```python
from build123d import *

# Parameters (mm, degrees)
BOSS_EXTRUDE1_DEPTH = 15
SKETCH2_R           = 7.5
CUT_EXTRUDE1_DEPTH  = 15
SKETCH3_R           = 20
BOSS_EXTRUDE2_DEPTH = 20
SKETCH4_R           = 10
CUT_EXTRUDE2_DEPTH  = 35


with BuildPart() as part:
    # Sketch1 → Boss-Extrude1 (new body)
    with BuildSketch(Plane.XY):
        with BuildLine():
            Line((-29.748120578, 3.87934557), (-24.393431116, 44.940897042))
            ThreePointArc((-24.393431116, 44.940897042), (-19.416464042, 54.272761237), (-9.519370827, 58.001224257))
            Line((-9.519370827, 58.001224257), (85, 58.001224257))
            ThreePointArc((85, 58.001224257), (99.971845495, 42.082615269), (83.166230421, 28.113736587))
            ThreePointArc((83.166230421, 28.113736587), (49.31881051, 20.091395843), (28.895124435, -8.066708368))
            ThreePointArc((28.895124435, -8.066708368), (-5.988234446, -29.396276095), (-29.748120578, 3.87934557))
        make_face()
    extrude(amount=BOSS_EXTRUDE1_DEPTH)

    # Sketch2 → Cut-Extrude1 (cut)
    with BuildSketch(Plane.XY.offset(15)):
        with Locations((-5, 39.686269666)):
            Circle(SKETCH2_R)
        with BuildLine():
            Line((85, 49.001224257), (45, 49.001224257))
            ThreePointArc((45, 49.001224257), (39, 43.001224257), (45, 37.001224257))
            Line((45, 37.001224257), (85, 37.001224257))
            ThreePointArc((85, 37.001224257), (91, 43.001224257), (85, 49.001224257))
        make_face()
    extrude(amount=-CUT_EXTRUDE1_DEPTH, mode=Mode.SUBTRACT)

    # Sketch3 → Boss-Extrude2 (add)
    with BuildSketch(Plane.XY.offset(15)):
        with Locations(Location((0, 0, 0), (0, 0, 180))):
            Circle(SKETCH3_R)
    extrude(amount=BOSS_EXTRUDE2_DEPTH)

    # Sketch4 → Cut-Extrude2 (cut)
    with BuildSketch(Plane.XY.offset(35)):
        Circle(SKETCH4_R)
    extrude(amount=-CUT_EXTRUDE2_DEPTH, mode=Mode.SUBTRACT)


solid = part.part
```
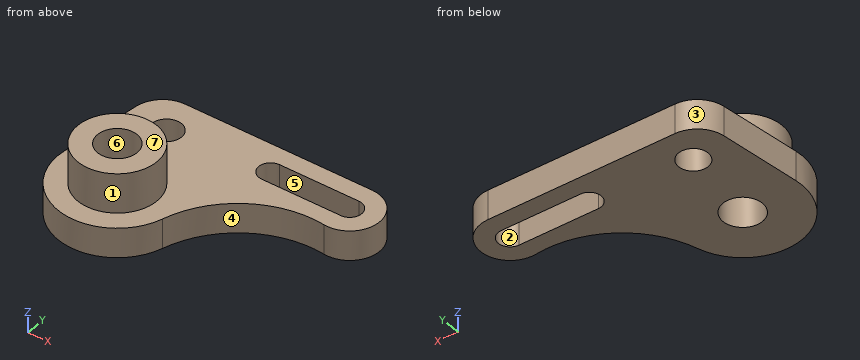
Geometry check sheet. Reference: the model listing, model coordinates, mm. Face numbers are marked on the shaded views. A direction names the side the tool comes from. Coordinates: 2 decimals unless noted, no trailing zeros. Order: outer loops, then holes, each group sorted by start corner. A loop starts at its lowest first (then second) coordinate and runs counter-clockwise, first axis right, second up. Notation, with made-up numbers: (4.25, -5.5) - (33.25, -5.5) arc R8 cw to (33.25, 1.5) - close; hole circle Ø10 at (60, 82.5). An arc over 180 degrees is marked (long way). Answer as a JSON object with one key per item and string values. Group by question number.
Item 1: Sectioned sample at C-C, the plane z = 5.5. Record the cut outline in (x, y).
Item 2: Sectioned sample at A-A, the plane x = 88.5. Record the cut outline in (y, z), and give its area (3 significant figures).
Item 3: Depth check by flat-ended pin: pin 1 Ø4 at (y, z) = (33.5, 8.5) entering from +X; pin 2 Ø12 at (x, y) = (82, 26.5) entering from +Z; pin 3 Ø3 at (x, z) = (-7, 20) entering from +Y; pin 4 Ø8 at (x, z) = (48, 16.5) entering from +Y. Enter the tip coordinate at first touch or a pass-through.
Item 4: Draft check along Y on the marked faces 4, 5, 6 and 7. Enter one of: +Y half, -Y half, draft (parallel to the pull), parting line (faces both ways), or undercut.
Item 5: Sectioned sample at D-D, the plane x = -5. Record the cut outline in (y, z), and give its area (3 significant figures).
Item 6: Tool access check on the marked faces 1, 2 and 3. Record the directions out of +Z, -Z, +X, -X, +Y, -Y that give a thin tool (end or side, any length) a straight path to the whole face; none if there is none.
Item 7: Sectioned sample at B-B, the plane y = -17. Record the cut outline in (x, z), and give its area (3 significant figures).
Item 8: Scan lines: probe 1 along Y at (x, z) = (0, 17); probe 2 along Y at (x, z) = (0, 12); probe 3 along X at (y, z) = (0.5, 27). Record each from-to range of solid material in increasing order.
Resolved:
{
 "1": {"outline": "(-29.75, 3.88) arc R30 ccw to (28.9, -8.07) arc R50 cw to (83.17, 28.11) arc R15 ccw (long way) to (85, 58) - (-9.52, 58) arc R15 ccw to (-24.39, 44.94) - close; hole circle Ø15 at (-5, 39.69); hole circle Ø20 at (0, 0); hole (45, 37) - (85, 37) arc R6 ccw to (85, 49) - (45, 49) arc R6 ccw to start"},
 "2": {"outline": "(28.42, 0) - (38.13, 0) - (38.13, 15) - (28.42, 15) - close; (47.87, 0) - (57.59, 0) - (57.59, 15) - (47.87, 15) - close", "area": "291 mm^2"},
 "3": {"pin 1": "x = 97.99", "pin 2": "z = 15", "pin 3": "y = 19.23", "pin 4": "y = 58"},
 "4": {"face 4": "-Y half", "face 5": "undercut", "face 6": "undercut", "face 7": "draft"},
 "5": {"outline": "(-29.58, 0) - (-8.66, 0) - (-8.66, 35) - (-19.36, 35) - (-19.36, 15) - (-29.58, 15) - close; (8.66, 0) - (32.19, 0) - (32.19, 15) - (19.36, 15) - (19.36, 35) - (8.66, 35) - close; (47.19, 0) - (58, 0) - (58, 15) - (47.19, 15) - close", "area": "1,260 mm^2"},
 "6": {"face 1": "+Z", "face 2": "+Z, -Z", "face 3": "+Z, -Z, -X, +Y"},
 "7": {"outline": "(-24.72, 0) - (24.72, 0) - (24.72, 15) - (10.54, 15) - (10.54, 35) - (-10.54, 35) - (-10.54, 15) - (-24.72, 15) - close", "area": "1,160 mm^2"},
 "8": {"probe 1": "-20 to -10, 10 to 20", "probe 2": "-30 to -10, 10 to 34.1, 45.28 to 58", "probe 3": "-19.99 to -9.99, 9.99 to 19.99"}
}
